from build123d import *

# Parameters (mm, degrees)
CROQUIS1_R              = 1.25
SALIENTE_EXTRUIR1_DEPTH = 15
CROQUIS5_R              = 11
CORTAR_EXTRUIR1_DEPTH   = 5
CROQUIS6_R              = 12.5
CORTAR_EXTRUIR2_DEPTH   = 5
CROQUIS4_R              = 22.5
CORTAR_EXTRUIR3_DEPTH   = 10


with BuildPart() as part:
    # Croquis1 → Saliente-Extruir1 (new body)
    with BuildSketch(Plane.XY):
        with BuildLine():
            ThreePointArc((0, 40), (-40, 0), (0, -40))
            Line((0, -40), (215, -50))
            ThreePointArc((215, -50), (265, 0), (215, 50))
            Line((215, 50), (0, 40))
        make_face()
        Circle(CROQUIS1_R, mode=Mode.SUBTRACT)
        with Locations((215, 0)):
            Circle(CROQUIS1_R, mode=Mode.SUBTRACT)
    extrude(amount=SALIENTE_EXTRUIR1_DEPTH)

    # Croquis5 → Cortar-Extruir1 (cut)
    with BuildSketch(Plane(origin=(0, 0, 0), x_dir=(-1, 0, 0), z_dir=(0, 0, -1))):
        Circle(CROQUIS5_R)
    extrude(amount=-CORTAR_EXTRUIR1_DEPTH, mode=Mode.SUBTRACT)

    # Croquis6 → Cortar-Extruir2 (cut)
    with BuildSketch(Plane.XY.offset(15)):
        with Locations((215, 0)):
            Circle(CROQUIS6_R)
    extrude(amount=-CORTAR_EXTRUIR2_DEPTH, mode=Mode.SUBTRACT)

    # Croquis4 → Cortar-Extruir3 (cut)
    with BuildSketch(Plane.XY.offset(15)):
        Circle(CROQUIS4_R)
    extrude(amount=-CORTAR_EXTRUIR3_DEPTH, mode=Mode.SUBTRACT)


solid = part.part
The model under review builds one solid part; all positions refer to its coordinate system, in mm. A direction names the side the tool comes from. Round coordinates to 2 decimals unless told otherwise and drop trailing zeros. Loops run counter-clockwise (first coordinate to the right, second up) from the corner with the lowest first, then second, coordinate; pieces in that order, holes last. Notation, with made-up numbers: (2, -13) -> (23, -13) arc R10 cw to (23, -9) -> close; hole circle Ø8 at (25.25, 37). An arc over 180 degrees is marked (long way). One line per question, with ' | ' between items. Start each with the question number.
Item 1: Add section D-D, the plane y = -43.5. Write out the cut boundary in (x, z).
Item 2: Wall thickness on line 1 along Y through (x, z) = (0, 3.8); line 2 along X through (y, z) = (-9, 11.5); line 3 along X through (y, z) = (-1, 5.5): over which ranges is each line inside the solid? List them lowest first. Write a range as [from, to].
Item 3: Add section C-C, the plane x = 50. Write out the cut boundary in (y, z).
Item 4: Add section B-B, the plane y = -15.5. Write out the cut boundary in (x, z), then the cut area to 3 significant figures.
Item 5: Add section A-A, the plane x = 19. Write out the cut boundary in (y, z), then the cut area to 3 significant figures.
Item 6: Draft analysis for pull direction Y (two halves, no side actions). For faces 3 (the face through (10.382, -19.961, 10.07)), 4 (the face through (110, 1, 15)), 5 (the face through (106, -44.93, 7.4)), state which applies: +Y half, -Y half, draft (parallel to the pull), parting line (faces both ways), or undercut.
Item 7: For pin 1 (13.5 mm diameter, centred on x = -3, y = -5.5, fed in from +Z); pin 2 (7.5 mm diameter, centred on x = 212.5, y = 2.5, fed in from +Z); pin 3 (3 mm diameter, centred on x = 103, z = 2.5, fed in from -Y), all flat-tipped, find the tip position at first contact; note any pin that passes through.
Item 8: Machinability: for faces 1 (the face through (10, 5, 5)), 2 (the face through (-39.99, 0.88, 7.4)), which of the approach directions +Z, -Z, +X, -X, +Y, -Y give a long, thin tool a straight path to every point of the face, cutting with its end or side? Answer none if there is none.
Return value:
1) outline: (75.25, 0) -> (239.65, 0) -> (239.65, 15) -> (75.25, 15) -> close
2) line 1: y = [-40, -11], [11, 40] | line 2: x = [-38.97, -20.62], [20.62, 206.33], [223.67, 264.18] | line 3: x = [-39.99, -22.48], [22.48, 214.25], [215.75, 264.99]
3) outline: (-42.33, 0) -> (42.33, 0) -> (42.33, 15) -> (-42.33, 15) -> close
4) outline: (-36.87, 0) -> (262.54, 0) -> (262.54, 15) -> (16.31, 15) -> (16.31, 5) -> (-16.31, 5) -> (-16.31, 15) -> (-36.87, 15) -> close | area: 4,160 mm2
5) outline: (-40.88, 0) -> (40.88, 0) -> (40.88, 15) -> (12.05, 15) -> (12.05, 5) -> (-12.05, 5) -> (-12.05, 15) -> (-40.88, 15) -> close | area: 985 mm2
6) face 3: undercut | face 4: draft | face 5: -Y half
7) pin 1: stops at z = 5 | pin 2: stops at z = 10 | pin 3: stops at y = -44.86
8) face 1: +Z | face 2: +Z, -Z, -X
